Model file for the job. Use its own axes, mm. Face numbers are marked on the shaded views. Round coordinates to 2 decimals unless told otherwise and drop trailing zeros. Order: outer loops, then holes, each group sorted by start corner. A loop starts at its lowest first (then second) coordinate and runs counter-clockwise, first axis right, second up. Notation, with made-up numbers: (24.25, 48) - (32.25, 48) arc R19 cw to (32.25, 71) - close; hole circle Ø6 at (35.25, -20.5). An arc over 180 degrees is marked (long way). Use one line per item in the form item = value.
from build123d import *

# Parameters (mm, degrees)
F0_W     = 152.4
F0_H     = 172.720005
F1_DEPTH = 101.6
F2_R     = 60.170779
F3_DEPTH = 101.601
F4_SIZE  = 5.08


with BuildPart() as f1:
    # F0 (on Front) → F1 (new body)
    with BuildSketch(Plane.XZ):
        with Locations((10.828421, 0.902369)):
            Rectangle(F0_W, F0_H)
    extrude(amount=F1_DEPTH)

    # F2 (on face) → F3 (cut, through all)
    with BuildSketch(Plane.XZ.offset(101.6)):
        with Locations((8.857357, 0)):
            Circle(F2_R)
    extrude(amount=-F3_DEPTH, mode=Mode.SUBTRACT)

    # F4
    f4_edges = [f1.edges().sort_by_distance(p)[0] for p in [
        (87.028421, -101.6, 0.90237),
        (10.828421, -101.6, 87.262372),
        (10.828421, -101.6, -85.457633),
        (-65.371579, -101.6, 0.90237),
        (10.828421, 0, -85.457633),
        (-65.371579, 0, 0.90237),
        (87.028421, 0, 0.90237),
        (10.828421, 0, 87.262372),
        (87.028421, -50.8, 87.262372),
    ]]
    chamfer(f4_edges, length=F4_SIZE)


solid = f1.part
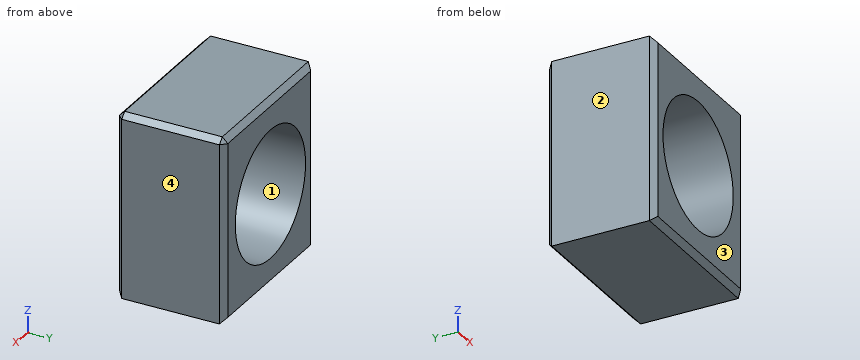
(1) Pull direction X, two halves, no side cores. Call the marked faces 1, 2, 3 and 4: released by +X, released by -X, zero draft, split by the parting line, or undercut.
Report:
face_1 = undercut
face_2 = released by -X
face_3 = zero draft
face_4 = released by +X
(2) Slice it at B-B on x = 42. Give the cut face in (y, z).
Report:
outline = (-101.6, -80.38) - (-96.52, -85.46) - (-5.08, -85.46) - (0, -80.38) - (0, -50.22) - (-101.6, -50.22) - close; (-101.6, 50.22) - (0, 50.22) - (0, 82.18) - (-5.08, 87.26) - (-96.52, 87.26) - (-101.6, 82.18) - close
(3) Slice it at C-C on y = -62. Give the cut face in (x, z).
Report:
outline = (-65.37, -85.46) - (87.03, -85.46) - (87.03, 82.18) - (81.95, 87.26) - (-65.37, 87.26) - close; hole circle Ø120.34 at (8.86, 0)
(4) Slice it at A-A on z = 48. Give the cut face in (x, y), then the cut area to 3 significant figures.
Report:
outline = (-65.37, -96.52) - (-60.29, -101.6) - (-27.43, -101.6) - (-27.43, 0) - (-60.29, 0) - (-65.37, -5.08) - close; (45.14, -101.6) - (81.95, -101.6) - (87.03, -96.52) - (87.03, -5.08) - (81.95, 0) - (45.14, 0) - close
area = 8,060 mm2
(5) Probe probe 1 along X at (y, z) = (-67, -28); probe 2 along X at (y, z) = (-95.5, 32.5); probe 3 along Z at (x, y) = (5, -27). List the from-to ranges inside material, lowest first. Write a range as [from, to].
Report:
probe_1 = [-65.37, -44.4], [62.12, 87.03]
probe_2 = [-65.37, -41.78], [59.5, 87.03]
probe_3 = [-85.46, -60.05], [60.05, 87.26]
